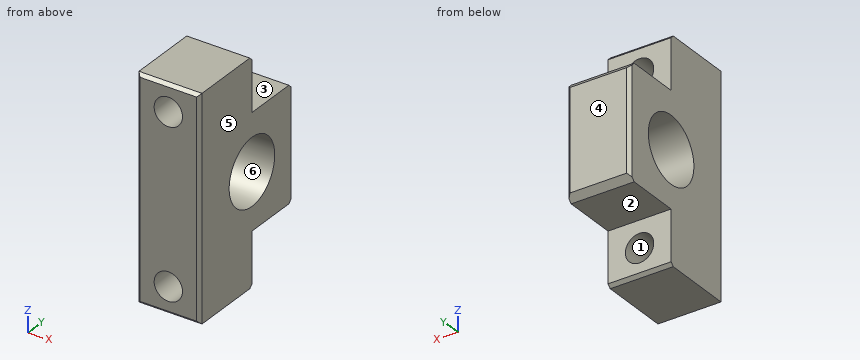
Autodesk Inventor part; units mm, degrees
ref_plane "YZ Plane" through (0, 0, 0) normal (1, 0, 0) x (0, 1, 0)
ref_plane "XZ Plane" through (0, 0, 0) normal (0, 1, 0) x (-1, 0, 0)
ref_plane "XY Plane" through (0, 0, 0) normal (0, 0, 1) x (1, 0, 0)
sketch "Sketch1" plane through (0, 0, 0) normal (1, 0, 0) x (0, 1, 0)
  line L0 (-24, 35) -> (24, 35)
  line L1 (24, 35) -> (24, -35)
  line L2 (24, -35) -> (-24, -35)
  line L3 (-24, -35) -> (-24, 35)
  line L4 (-24, 35) -> (24, -35) construction
  line L5 (24, 35) -> (-24, -35) construction
  line L6 (-43, 18) -> (43, 18)
  line L7 (43, 18) -> (43, -18)
  line L8 (43, -18) -> (-43, -18)
  line L9 (-43, -18) -> (-43, 18)
  line L10 (-43, 18) -> (43, -18) construction
  line L11 (43, 18) -> (-43, -18) construction
  circle A0 centre (24, 0) radius 10.5
  line L12 (0, 35) -> (0, -35)
  point P0 (0, 0)
  point P1 (24, -18)
  point P2 (24, 18)
  dimension "d0" = 36
  dimension "d1" = 70
  dimension "d2" = 19
  dimension "d3" = 24
  dimension "d4" = 21
extrude "Extrusion1" add sketch "Sketch1" along normal mid plane 20 contours L0 L1 L6 L12 | L6 L1 A0 L8 L12 | L6 L7 L8 L1 A0 | L8 L1 L2 L12
sketch "Sketch2" plane through (-10, 24, -18) normal (0, 1, 0) x (1, 0, 0)
  line L0 (0, 0) -> (20, 0)
  line L1 (20, 17) -> (20, 0)
  line L2 (0, 17) -> (20, 17)
  line L3 (0, 0) -> (0, 17)
  line L4 (0, -53) -> (20, -53)
  line L5 (20, -36) -> (20, -53)
  line L6 (0, -36) -> (20, -36)
  line L7 (0, -53) -> (0, -36)
  line L8 (0, -53) -> (20, -36)
  line L9 (20, 17) -> (20, 0)
  line L10 (20, 0) -> (0, 17)
  point P0 (10, -18)
  point P1 (10, -44.5)
  point P2 (10, 8.5)
hole "Hole1" at (0, 24, 26.5) at (0, 24, -26.5) direction (0, -1, 0) diameter 9 end through all
chamfer "Chamfer1" distance 1 angle 45 2 edges at (-10, 43, 0) (10, 43, 0)
chamfer "Chamfer2" distance 1 angle 45 6 edges at (0, 24, 35) (0, 24, -35) (-10, 0, 0) (0, 0, -35) (10, 0, 0) (0, 0, 35)
chamfer "Chamfer3" distance 2 angle 45 2 edges at (0, 43, -18) (0, 43, 18)
properties part number "Goi_do_A" material "Iron, Gray"
Verification items for the finished model (mm, model axes). Face numbers are marked on the shaded views. A direction names the side the tool comes from. Round coordinates to 2 decimals unless told otherwise and drop trailing zeros. Order: outer loops, then holes, each group sorted by start corner. A loop starts at its lowest first (then second) coordinate and runs counter-clockwise, first axis right, second up. Notation, with made-up numbers: (-21.5, 45.5) -> (30.5, 45.5) arc R26 ccw to (30.5, 69.5) -> close; hole circle Ø5 at (7, 21.5). An arc over 180 degrees is marked (long way). Put each result on its own line as item: value. Start each with the question number.
(1) Section check A-A (x = 0). Enter the section's corners in (y, z).
(2) Section check C-C (z = 26.5). Enter the section's corners in (x, y), then the cut area to 3 significant figures.
(3) Section check B-B (y = 19). Enter the section's corners in (x, z).
(4) Tool access check on the marked faces 1, 2 and 3. Record the directions out of +Z, -Z, +X, -X, +Y, -Y that give a thin tool (end or side, any length) a straight path to the whole face; none if there is none.
(5) Section check D-D (y = 30). Enter the section's corners in (x, z).
(6) Material ranges on line 1 along Y through (x, z) = (0, 0); line 2 along X through (y, z) = (6, 26.5); line 3 along Z through (x, y) = (0, 18.5), recorded low to high.
(7) Draft check along Y on the marked faces 4, 5 and 6. Enter one of: +Y half, -Y half, draft (parallel to the pull), parting line (faces both ways), or undercut.
(8) Depth check by flat-ended pin: pin 1 Ø8 at (x, z) = (0.5, -25) entering from +Y; pin 2 Ø5 at (x, y) = (-5, 33) entering from -Z; pin 3 Ø5 at (x, y) = (6, 28.5) entering from +Z. Enter the tip coordinate at first touch or a pass-through.
Completed:
1. outline: (0, -34) -> (1, -35) -> (23, -35) -> (24, -34) -> (24, -31) -> (0, -31) -> close; (0, -22) -> (24, -22) -> (24, -18) -> (41, -18) -> (43, -16) -> (43, 16) -> (41, 18) -> (24, 18) -> (24, 22) -> (0, 22) -> close; (0, 31) -> (24, 31) -> (24, 34) -> (23, 35) -> (1, 35) -> (0, 34) -> close; hole circle Ø21 at (24, 0)
2. outline: (-10, 1) -> (-9, 0) -> (-4.5, 0) -> (-4.5, 24) -> (-10, 24) -> close; (4.5, 0) -> (9, 0) -> (10, 1) -> (10, 24) -> (4.5, 24) -> close
2. area: 263 mm2
3. outline: (-10, -35) -> (10, -35) -> (10, -9.23) -> (-10, -9.23) -> close; (-10, 9.23) -> (10, 9.23) -> (10, 35) -> (-10, 35) -> close; hole circle Ø9 at (0, -26.5); hole circle Ø9 at (0, 26.5)
4. face 1: +Y, -Y
4. face 2: -Z, +X, -X, +Y
4. face 3: +Z, +X, -X, +Y
5. outline: (-10, -18) -> (10, -18) -> (10, -8.62) -> (-10, -8.62) -> close; (-10, 8.62) -> (10, 8.62) -> (10, 18) -> (-10, 18) -> close
6. line 1: y = 0 to 13.5, 34.5 to 43
6. line 2: x = -10 to -4.5, 4.5 to 10
6. line 3: z = -35 to -31, -22 to -8.94, 8.94 to 22, 31 to 35
7. face 4: +Y half
7. face 5: draft
7. face 6: undercut
8. pin 1: stops at y = 24
8. pin 2: stops at z = -18
8. pin 3: stops at z = 18
